Input: part model. Units: mm. Frame: model coordinates. A direction names the side the tool comes from. Round coordinates to 2 decimals unless told otherwise and drop trailing zeros. Loops run counter-clockwise (first coordinate to the right, second up) from the corner with the lowest first, then second, coordinate; pieces in that order, holes last. Notation, with made-up numbers: (57.5, 49.25) -> (115.5, 49.25) arc R12 ccw to (115.5, 63.25) -> close; hole circle Ø6 at (55, -39). An arc over 180 degrees is marked (long way). Answer as a JSON object with one key per item and string values.
Autodesk Inventor part; units mm, degrees
ref_plane "YZ Plane" through (0, 0, 0) normal (1, 0, 0) x (0, 1, 0)
ref_plane "XZ Plane" through (0, 0, 0) normal (0, 1, 0) x (-1, 0, 0)
ref_plane "XY Plane" through (0, 0, 0) normal (0, 0, 1) x (1, 0, 0)
sketch "Skizze1" plane through (0, 0, 0) normal (1, 0, 0) x (0, 1, 0)
  arc A0 (11.0636, -2.8051) -> (10.5724, 2.9449) centre (10, 0) ccw
  line L0 (11.0636, -2.8051) -> (0, -7)
  line L1 (0, -7) -> (0, 5)
  line L2 (0, 5) -> (10.5724, 2.9449)
  point P0 (0, 0)
  dimension "d0" = 3
  dimension "d1" = 10
  dimension "d2" = 12
  dimension "d3" = 5
extrude "Extrusion1" add sketch "Skizze1" along normal mid plane 2
sketch "Skizze2" plane through (0, 0, 0) normal (0, 1, 0) x (-1, 0, 0)
  line L0 (-1, 2.9449) -> (-1, 5)
  line L1 (-1, 5) -> (4, 5)
  line L2 (4, 5) -> (4, -7)
  line L3 (4, -7) -> (-1, -7)
  line L4 (-1, -7) -> (-1, 5)
  line L5 (1, -7) -> (-1, -7)
  point P0 (0, 0)
  point P1 (-1, 2.9449)
  dimension "d6" = 5
extrude "Extrusion2" add sketch "Skizze2" against normal blind 2
fillet "Rundung1" radius 2 1 edges at (-1, 0, -1)
sketch "Skizze3" plane through (1, 0, 0) normal (1, 0, 0) x (0, 0, -1)
  arc A0 (2.8051, 11.0636) -> (-2.9449, 10.5724) centre (0, 10) ccw
  circle A1 centre (0, 10) radius 1
  line L0 (0, 10) -> (0, -2) construction
  line L1 (7, -2) -> (-5, -2)
  circle A2 centre (0, 6) radius 1
  point P0 (0, 0)
  dimension "d10" = 2
  dimension "d13" = 4
extrude "Extrusion3" cut sketch "Skizze3" against normal blind 4.75
properties part number "P_Wing_aileron_lever"
1) Section B-B, the plane y = 10. Output: boundary loops of the cut face in (x, z).
Output:
{"outline": "(-1, -3.21) -> (1, -3.21) -> (1, -1) -> (-1, -1) -> close; (-1, 1) -> (1, 1) -> (1, 3.06) -> (-1, 3.06) -> close"}
2) Contact query for flat-ended pins moving along their axis: P1, Ø0.5, axis at x = -3.5, z = 2, coming from the +Y side; P2, Ø2, axis at x = 0, z = 3, coming from the +Y side; P3, Ø3, axis at y = 8, z = -4.5, coming from the -X side. Output: stop coordinate, or through.
Output:
{"P1": "stops at y = 0", "P2": "stops at y = 12.24", "P3": "stops at x = -1"}
3) Reachability of faces 4 (the face through (-1, -2, -1)), 5 (the face through (-3.5, 0, -0.9)) from +Z, -Z, +X, -X, +Y, -Y: full face, straight path, thin tool, end or side. Return the list, or none.
Output:
{"face 4": "+Z, -Z, +X, -X, -Y", "face 5": "+Z, -Z, -X, +Y"}
4) Draft query along Y for faces 1 (the face through (-0.139, 5.212, 3.987)), 2 (the face through (0, 11, 0)), 3 (the face through (-1, -1, 5)). Return one class per face: +Y half, -Y half, draft (parallel to the pull), parting line (faces both ways), or undercut.
Output:
{"face 1": "+Y half", "face 2": "undercut", "face 3": "draft"}
5) Section A-A, the plane x = -0.25. Output: boundary loops of the cut face in (y, z), plus the area to 3 significant figures.
Output:
{"outline": "(-2, -7) -> (0, -7) -> (11.06, -2.81) arc R3 ccw to (10.57, 2.94) -> (0, 5) -> (-2, 5) -> close; hole circle Ø2 at (6, 0); hole circle Ø2 at (10, 0)", "area": "123 mm^2"}
6) Section D-D, the plane z = -1.75. Output: boundary loops of the cut face in (x, y).
Output:
{"outline": "(-4, -2) -> (1, -2) -> (1, 12.44) -> (-1, 12.44) -> (-1, 2) arc R2 cw to (-3, 0) -> (-4, 0) -> close"}
7) Section C-C, the plane z = 0. Output: boundary loops of the cut face in (x, y), plus the area to 3 significant figures.
Output:
{"outline": "(-4, -2) -> (1, -2) -> (1, 5) -> (-1, 5) -> (-1, 2) arc R2 cw to (-3, 0) -> (-4, 0) -> close; (-1, 7) -> (1, 7) -> (1, 9) -> (-1, 9) -> close; (-1, 11) -> (1, 11) -> (1, 13) -> (-1, 13) -> close", "area": "28.9 mm^2"}
8) Ray query, probe 1 along Y at (x, z) = (0.1, 0); probe 2 along Y at (x, z) = (-3.25, 4.5); probe 3 along X at (y, z) = (4.5, 0). Return the intervals inside material, ascending.
Output:
{"probe 1": "y = -2 to 5, 7 to 9, 11 to 13", "probe 2": "y = -2 to 0", "probe 3": "x = -1 to 1"}
